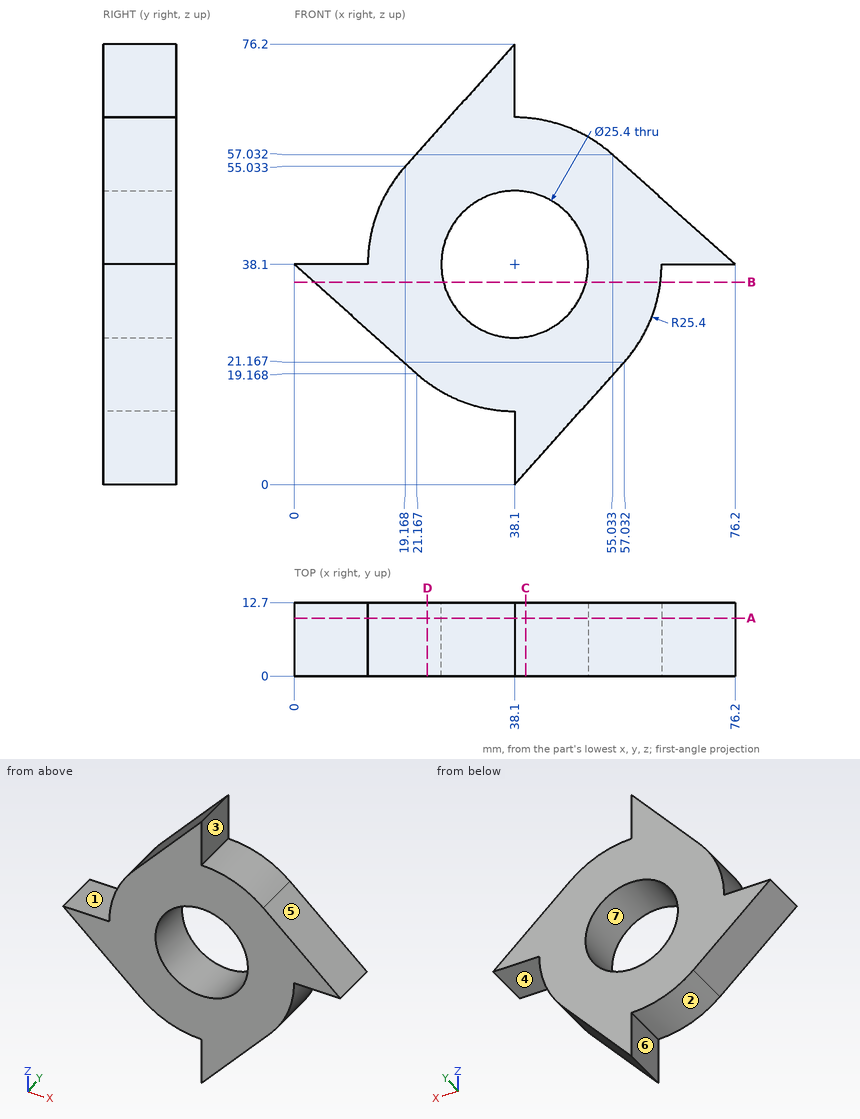
Here's the drawing with two shaded views (mm, measured from the low corner). I have some questions. A direction names the side the tool comes from. Give positions to 0.01 mm unless a question says otherwise; leave off trailing zeros. Loops run counter-clockwise (first coordinate to the right, second up) from the corner with the lowest first, then second, coordinate; pieces in that order, holes last. Notation, with made-up numbers: (76.5, 5.25) -> (123.5, 5.25) arc R28 cw to (123.5, 32.25) -> close; hole circle Ø4 at (48, -7). An arc over 180 degrees is marked (long way). Answer as a JSON object with one key per item and string values. Group by question number.
Item 1: Imagine slicing it at D-D on x = 23. Write out the boundary of the cut face in (y, z).
Item 2: Imagine slicing it at C-C on x = 40. Write out the boundary of the cut face in (y, z), then the cut area to 3 significant figures.
Item 3: Imagine slicing it at A-A on y = 10. Write out the boundary of the cut face in (x, z), then the cut area to 3 significant figures.
Item 4: Thinking about a two-plate mould opening in X: for the marked faces 4, 5, 6 and 7, which applies, pulls with the +X half, pulls with the -X half, needs draft (parallel to the pull), parting line crosses it, or undercut?
Item 5: I need wall thicknesses on L1, parallel to X at y = 8.25, z = 32 (1 decimal); L2, parallel to Z at x = 44, y = 7.5 (1 decimal); L3, parallel to Z at x = 51, y = 9.75. Which ranges of each line are inside material? Lowest first, please.
Item 6: On a 3-axis mill with a long thin cutter (end or side, diameter ignored), from which of +Z, -Z, +X, -X, +Y, -Y can I reach the whole of each face in a straight line? I mean the marked faces 1, 2 and 3. Say none if no direction works.
Item 7: Imagine slicing it at B-B on z = 35. Write out the boundary of the cut face in (x, y).
Item 8: Will these pins go through, and if not, where does the flat tip stop? pin 1 (3 mm diameter, centred on y = 10.5, z = 55, fed in from -X); pin 2 (1.5 mm diameter, centred on x = 39, y = 8, fed in from -Z); pin 3 (4 mm diameter, centred on y = 9, z = 13, fed in from +X).
Answer list:
{
 "1": {"outline": "(0, 17.68) -> (12.7, 17.68) -> (12.7, 59.32) -> (0, 59.32) -> close"},
 "2": {"outline": "(0, 2.12) -> (12.7, 2.12) -> (12.7, 25.54) -> (0, 25.54) -> close; (0, 50.66) -> (12.7, 50.66) -> (12.7, 63.43) -> (0, 63.43) -> close", "area": "460 mm2"},
 "3": {"outline": "(0, 38.1) -> (21.17, 19.17) arc R25.4 ccw to (38.1, 12.7) -> (38.1, 0) -> (57.03, 21.17) arc R25.4 ccw to (63.5, 38.1) -> (76.2, 38.1) -> (55.03, 57.03) arc R25.4 ccw to (38.1, 63.5) -> (38.1, 76.2) -> (19.17, 55.03) arc R25.4 ccw to (12.7, 38.1) -> close; hole circle Ø25.4 at (38.1, 38.1)", "area": "1,880 mm2"},
 "4": {"face 4": "needs draft", "face 5": "pulls with the +X half", "face 6": "pulls with the -X half", "face 7": "undercut"},
 "5": {"L1": "x = 6.8 to 27, 49.2 to 62.8", "L2": "z = 6.6 to 26.9, 49.3 to 62.8", "L3": "z = 14.42 to 59.98"},
 "6": {"face 1": "+Z, -X, +Y, -Y", "face 2": "-Z, -X, +Y, -Y", "face 3": "+Z, +X, +Y, -Y"},
 "7": {"outline": "(3.47, 0) -> (25.78, 0) -> (25.78, 12.7) -> (3.47, 12.7) -> close; (50.42, 0) -> (63.31, 0) -> (63.31, 12.7) -> (50.42, 12.7) -> close"},
 "8": {"pin 1": "stops at x = 17.9", "pin 2": "stops at z = 0.17", "pin 3": "stops at x = 51.52"}
}
